from build123d import *

# Parameters (mm, degrees)
F0_W     = 36.9340777397
F0_H     = 34.6101336181
F1_DEPTH = 30
F2_R     = 5.08
F3_T     = -2.54


# Not quite as in the source:
# - a shell that OpenCascade refuses in one call is made with other operations: the cavity is built on its own and cut out


with BuildPart() as f1:
    # F0 (on Top) → F1 (new body)
    with BuildSketch(Plane.XY):
        with Locations((18.4670388699, -17.3050668091)):
            Rectangle(F0_W, F0_H)
    extrude(amount=F1_DEPTH)

    # F2
    f2_edges = [f1.edges().sort_by_distance(p)[0] for p in [
        (36.934078, -34.610134, 15),
        (36.934078, 0, 15),
        (36.934078, -17.305067, 0),
        (18.467039, -34.610134, 0),
        (0, -17.305067, 0),
        (18.467039, 0, 0),
        (18.467039, 0, 30),
        (36.934078, -17.305067, 30),
        (18.467039, -34.610134, 30),
        (0, -34.610134, 15),
        (0, -17.305067, 30),
        (0, 0, 15),
    ]]
    fillet(f2_edges, radius=F2_R)

    # F3: a shell. OpenCascade refuses it in one call, so the cavity is built on its own and cut out:
    # the body offset inwards by the wall thickness, plus a prism from it out through each open face.
    f3_core = offset(f1.part, amount=F3_T, mode=Mode.PRIVATE)
    f3_exits = [f3_core.faces().sort_by_distance(p)[0] for p in [
        (18.467039, -17.305067, 27.46),
        (18.467039, -32.070134, 15),
        (18.467039, -2.54, 15),
        (2.54, -17.305067, 15),
        (18.467039, -17.305067, 2.54),
        (34.394078, -17.305067, 15),
    ]]
    add(f3_core, mode=Mode.SUBTRACT)
    extrude(f3_exits, amount=-F3_T, mode=Mode.SUBTRACT)


solid = f1.part
The model under review builds one solid part; all positions refer to its coordinate system, in mm. A direction names the side the tool comes from. Round coordinates to 2 decimals unless told otherwise and drop trailing zeros. Write each loop counter-clockwise with the first axis right and the second up, starting at its lowest first coordinate (ties: lowest second). Pieces come first, ordered by that corner, then holes. Notation, with made-up numbers: (75.25, -27) -> (100.25, -27) arc R31 ccw to (100.25, 1) -> close; hole circle Ø6 at (68, 30). An arc over 180 degrees is marked (long way). Answer as a JSON object with one key per item and string values.
1. Clearance check with flat-ended pins moving along their axes: pin 1 (1.3 mm diameter, centred on x = 21, y = -34, fed in from +Z); pin 2 (0.8 mm diameter, centred on y = -33.5, z = 13, fed in from +X); pin 3 (1.3 mm diameter, centred on x = 14, y = -1, fed in from +Z); pin 4 (8 mm diameter, centred on x = 13.5, y = -29, fed in from -Z). State where each tip first meets the part, or that it passes through.
Results found:
{"pin 1": "stops at z = 28.27", "pin 2": "stops at x = 35.47", "pin 3": "stops at z = 28.67", "pin 4": "stops at z = 0"}
2. We need section C-C on y = -31. State the section outline as (x, z) points.
Results found:
{"outline": "(0.22, 5.08) arc R4.86 ccw to (5.08, 0.22) -> (31.85, 0.22) arc R4.86 ccw to (36.72, 5.08) -> (36.72, 24.92) arc R4.86 ccw to (31.85, 29.78) -> (5.08, 29.78) arc R4.86 ccw to (0.22, 24.92) -> close; hole (3.01, 5.08) arc R2.07 ccw to (5.08, 3.01) -> (31.85, 3.01) arc R2.07 ccw to (33.93, 5.08) -> (33.93, 24.92) arc R2.07 ccw to (31.85, 26.99) -> (5.08, 26.99) arc R2.07 ccw to (3.01, 24.92) -> close"}
3. The part is to be moulded in two halves that separate along Z. For faces 1 (the face through (18.654, -33.162, 1.528)), 2 (the face through (36, -29.53, 15)), 3 (the face through (35.49, -17.13, 28.47)), say which applies: pulls with the +Z half, pulls with the -Z half, needs draft (parallel to the pull), parting line crosses it, or undercut.
Results found:
{"face 1": "pulls with the -Z half", "face 2": "undercut", "face 3": "pulls with the +Z half"}
4. We need section B-B on x = 29.5. State the section outline as (y, z) points, and give its area (3 significant figures).
Results found:
{"outline": "(-34.61, 5.08) arc R5.08 ccw to (-29.53, 0) -> (-29.53, 2.54) arc R2.54 cw to (-32.07, 5.08) -> close; (-34.61, 24.92) -> (-32.07, 24.92) arc R2.54 cw to (-29.53, 27.46) -> (-29.53, 30) arc R5.08 ccw to start; (-5.08, 0) arc R5.08 ccw to (0, 5.08) -> (-2.54, 5.08) arc R2.54 cw to (-5.08, 2.54) -> close; (-5.08, 27.46) arc R2.54 cw to (-2.54, 24.92) -> (0, 24.92) arc R5.08 ccw to (-5.08, 30) -> close", "area": "60.8 mm^2"}
5. We need section A-A on z = 13.75. State the section outline as (x, y) points.
Results found:
{"outline": "(0, -29.53) arc R5.08 ccw to (5.08, -34.61) -> (5.08, -32.07) arc R2.54 cw to (2.54, -29.53) -> close; (0, -5.08) -> (2.54, -5.08) arc R2.54 cw to (5.08, -2.54) -> (5.08, 0) arc R5.08 ccw to start; (31.85, -34.61) arc R5.08 ccw to (36.93, -29.53) -> (34.39, -29.53) arc R2.54 cw to (31.85, -32.07) -> close; (31.85, -2.54) arc R2.54 cw to (34.39, -5.08) -> (36.93, -5.08) arc R5.08 ccw to (31.85, 0) -> close"}
6. We need section D-D on z = 25.5. State the section outline as (x, y) points, and give its area (3 significant figures).
Results found:
{"outline": "(0.03, -29.53) arc R5.05 ccw to (5.08, -34.58) -> (31.85, -34.58) arc R5.05 ccw to (36.9, -29.53) -> (36.9, -5.08) arc R5.05 ccw to (31.85, -0.03) -> (5.08, -0.03) arc R5.05 ccw to (0.03, -5.08) -> close; hole (2.61, -29.53) arc R2.47 ccw to (5.08, -32) -> (31.85, -32) arc R2.47 ccw to (34.33, -29.53) -> (34.33, -5.08) arc R2.47 ccw to (31.85, -2.61) -> (5.08, -2.61) arc R2.47 ccw to (2.61, -5.08) -> close", "area": "324 mm^2"}
7. To check wall thickness, follow line 1 along Z through (x, y) = (33, -11); line 2 along Y through (x, z) = (21, 2.5); line 3 along Y through (x, z) = (32.5, 14.5). State the ranges of each line that lie inside material, in increasing order.
Results found:
{"line 1": "z = 0.13 to 2.81, 27.19 to 29.87", "line 2": "y = -33.91 to -29.53, -5.08 to -0.7", "line 3": "y = -34.57 to -31.99, -2.62 to -0.04"}
8. Machinability: for faces 4 (the face through (5.08, -1, 15)), 5 (the face through (18.654, -3.264, 3.304)), 6 (the face through (18, -29.53, 29)), 7 (the face through (1.449, -17.134, 28.472)), 8 (the face through (36, -5.08, 15)), which of the approach directions +Z, -Z, +X, -X, +Y, -Y give a long, thin tool a straight path to every point of the face, cutting with its end or side? Answer none if there is none.
Results found:
{"face 4": "+Y, -Y", "face 5": "none", "face 6": "+Z, -Z", "face 7": "+Z, -X, +Y, -Y", "face 8": "+X, -X"}
